```python
from build123d import *

# Parameters (mm, degrees)
EXTRUDE_1_DEPTH          = 1.6
SKETCH_2_R               = 1.1
CUT_EXTRUDE_1_DEPTH      = 40.983559121
FILLET_1_R               = 1
SKETCH_4_W               = 6.5
SKETCH_4_H               = 6.5
CUT_EXTRUDE_2_DEPTH      = 40.983559121
FILLET_2_R               = 1
SKETCH_8_W               = 28.8
SKETCH_8_H               = 14.3
CUT_EXTRUDE_3_DEPTH      = 1.6
EXTRUDE_START            = -1.75
EXTRUDE_2_DEPTH          = 26.9
CUT_EXTRUDE_4_DEPTH      = 42.601502377
CUT_EXTRUDE_4_DEPTH_BACK = 42.601502377
CUT_EXTRUDE_6_DEPTH      = 42.18403817
SHELL_START              = -28.2
SHELL_3_DEPTH            = 23.3
SHELL_START_2            = -2.83732082
SHELL_3_2_DEPTH          = 1.8
FILLET_3_R               = 3
SKETCH_15_R              = 3.1
CUT_EXTRUDE_8_DEPTH      = 1.8
FILLET_5_R               = 2
CUT_EXTRUDE_9_DEPTH      = 42.18403817
CUT_EXTRUDE_START        = -1.8
CUT_EXTRUDE_10_DEPTH     = 1.8


with BuildPart() as part:
    # 草图1 → 凸台-拉伸1 (new body)
    with BuildSketch(Plane(origin=(0, 0, 0), x_dir=(1, 0, 0), z_dir=(0, 1, 0))):
        with BuildLine():
            Line((-24.25, 8.5), (-19, 8.5))
            Line((-19, 8.5), (-19, -8.5))
            Line((-19, -8.5), (-24.25, -8.5))
            Line((-24.25, -8.5), (-24.25, -28.75))
            ThreePointArc((-24.25, -28.75), (-23.371320344, -30.871320344), (-21.25, -31.75))
            Line((-21.25, -31.75), (21.25, -31.75))
            ThreePointArc((21.25, -31.75), (23.371320344, -30.871320344), (24.25, -28.75))
            Line((24.25, -28.75), (24.25, -8.5))
            Line((24.25, -8.5), (19, -8.5))
            Line((19, -8.5), (19, 8.5))
            Line((19, 8.5), (24.25, 8.5))
            Line((24.25, 8.5), (24.25, 28.75))
            ThreePointArc((24.25, 28.75), (23.371320344, 30.871320344), (21.25, 31.75))
            Line((21.25, 31.75), (-21.25, 31.75))
            ThreePointArc((-21.25, 31.75), (-23.371320344, 30.871320344), (-24.25, 28.75))
            Line((-24.25, 28.75), (-24.25, 8.5))
        make_face()
    extrude(amount=EXTRUDE_1_DEPTH)

    # 草图2 → 切除-拉伸1 (cut, through all)
    with BuildSketch(Plane(origin=(0, 1.6, 0), x_dir=(1, 0, 0), z_dir=(0, 1, 0))):
        with Locations(Location((-19.9, 27.9, 0), (0, 0, 270))):
            Circle(SKETCH_2_R)
        with Locations(Location((19.9, 27.9, 0), (0, 0, 90))):
            Circle(SKETCH_2_R)
        with Locations(Location((19.9, -27.9, 0), (0, 0, 270))):
            Circle(SKETCH_2_R)
        with Locations(Location((-19.9, -27.9, 0), (0, 0, 90))):
            Circle(SKETCH_2_R)
    extrude(amount=-CUT_EXTRUDE_1_DEPTH, mode=Mode.SUBTRACT)

    # 圆角1
    fillet_1_edges = [part.edges().sort_by_distance(p)[0] for p in [
        (19, 0.8, -8.5),
        (19, 0.8, 8.5),
        (-19, 0.8, 8.5),
        (-19, 0.8, -8.5),
    ]]
    fillet(fillet_1_edges, radius=FILLET_1_R)

    # 草图4 → 切除-拉伸2 (cut, through all)
    with BuildSketch(Plane(origin=(0, 1.6, 0), x_dir=(1, 0, 0), z_dir=(0, 1, 0))):
        with Locations((-6, -18.75)):
            Rectangle(SKETCH_4_W, SKETCH_4_H)
        with Locations((6, -18.75)):
            Rectangle(SKETCH_4_W, SKETCH_4_H)
    extrude(amount=-CUT_EXTRUDE_2_DEPTH, mode=Mode.SUBTRACT)

    # 圆角2
    fillet_2_edges = [part.edges().sort_by_distance(p)[0] for p in [
        (-2.75, 0.8, 15.5),
        (-2.75, 0.8, 22),
        (9.25, 0.8, 15.5),
        (9.25, 0.8, 22),
        (2.75, 0.8, 22),
        (2.75, 0.8, 15.5),
        (-9.25, 0.8, 22),
        (-9.25, 0.8, 15.5),
    ]]
    fillet(fillet_2_edges, radius=FILLET_2_R)

    # 草图8 → 切除-拉伸3 (cut)
    with BuildSketch(Plane(origin=(0, 1.6, 0), x_dir=(1, 0, 0), z_dir=(0, 1, 0))):
        with Locations((0, -5.55)):
            Rectangle(SKETCH_8_W, SKETCH_8_H)
    extrude(amount=-CUT_EXTRUDE_3_DEPTH, mode=Mode.SUBTRACT)

    # 草图10 → 凸台-拉伸2 (add)
    with BuildSketch(Plane(origin=(0, 0, -31.75), x_dir=(-1, 0, 0), z_dir=(0, 0, -1)).offset(EXTRUDE_START)):
        Polygon((-9, 1.6), (9, 1.6), (7, 11.6), (-7, 11.6), align=None)
    extrude(amount=-EXTRUDE_2_DEPTH)

    # 草图11 → 切除-拉伸4 (cut, two sides: drawn at the far end of the back side and taken through both)
    with BuildSketch(Plane(origin=(0, 0, 0), x_dir=(0, 0, -1), z_dir=(1, 0, 0)).offset(-CUT_EXTRUDE_4_DEPTH_BACK)):
        Polygon((6.1, 11.6), (3.1, 4.6), (3.1, 11.6), align=None)
    extrude(amount=CUT_EXTRUDE_4_DEPTH + CUT_EXTRUDE_4_DEPTH_BACK, mode=Mode.SUBTRACT)

    # 草图14 → 切除-拉伸6 (cut, through all)
    with BuildSketch(Plane(origin=(0, 1.6, 0), x_dir=(1, 0, 0), z_dir=(0, 1, 0))):
        Polygon((-9, 30), (9, 30), (11.5, 31.75), (-11.5, 31.75), align=None)
    extrude(amount=-CUT_EXTRUDE_6_DEPTH, mode=Mode.SUBTRACT)

    # 抽壳3: read off the stored shape, not the designer's step
    # 抽壳3 outline → 抽壳3 (cut)
    with BuildSketch(Plane.XY.offset(SHELL_START)):
        Polygon((-7.484352975, 0), (7.484352975, 0), (5.524352975, 9.8), (-5.524352975, 9.8), align=None)
    extrude(amount=SHELL_3_DEPTH, mode=Mode.SUBTRACT)

    # Shell 3 2 outline → Shell 3 2 (add)
    with BuildSketch(Plane(origin=(0, 0, 0), x_dir=(1, 0, 0), z_dir=(0, 0.3939192985791679, 0.9191450300180578)).offset(SHELL_START_2)):
        Polygon((6.638245748, 5.818680827), (5.524352975, 11.878076985), (-5.524352975, 11.878076985), (-6.638245748, 5.818680827), align=None)
    extrude(amount=SHELL_3_2_DEPTH)

    # 圆角3
    fillet_3_edges = [part.edges().sort_by_distance(p)[0] for p in [
        (-11.5, 0.8, -31.75),
        (11.5, 0.8, -31.75),
        (9, 0.8, -30),
        (-9, 0.8, -30),
    ]]
    fillet(fillet_3_edges, radius=FILLET_3_R)

    # 草图15 → 切除-拉伸8 (cut)
    with BuildSketch(Plane(origin=(0, 0, -30), x_dir=(-1, 0, 0), z_dir=(0, 0, -1))):
        with Locations((0, 5.1)):
            Circle(SKETCH_15_R)
    extrude(amount=-CUT_EXTRUDE_8_DEPTH, mode=Mode.SUBTRACT)

    # 圆角5
    fillet_5_edges = [part.edges().sort_by_distance(p)[0] for p in [
        (9, 1.6, -16.626473173),
        (-9, 1.6, -16.626473173),
        (7, 11.6, -18.05),
        (-7, 11.6, -18.05),
    ]]
    fillet(fillet_5_edges, radius=FILLET_5_R)

    # 草图16 → 切除-拉伸9 (cut, through all)
    with BuildSketch(Plane(origin=(0, 1.6, 0), x_dir=(1, 0, 0), z_dir=(0, 1, 0))):
        Polygon((-11.839607805, 25.75), (-11.839607805, 28.75), (-16.839607805, 22.75), (-16.839607805, 19.75), align=None)
        Polygon((-11.839607805, 20.75), (-11.839607805, 23.75), (-16.839607805, 17.75), (-16.839607805, 14.75), align=None)
        Polygon((-11.839607805, 15.75), (-11.839607805, 18.75), (-16.839607805, 12.75), (-16.839607805, 9.75), align=None)
        Polygon((-11.839607805, 10.75), (-11.839607805, 13.75), (-16.839607805, 7.75), (-16.839607805, 4.75), align=None)
    cut_extrude_9 = extrude(amount=-CUT_EXTRUDE_9_DEPTH, mode=Mode.SUBTRACT)

    # 镜向1: 切除-拉伸9 across plane
    add(cut_extrude_9.mirror(Plane(origin=(0, 0, 0), x_dir=(0, 0, 1), z_dir=(1, 0, 0))), mode=Mode.SUBTRACT)

    # 草图18 → 切除-拉伸10 (cut)
    with BuildSketch(Plane(origin=(-8.961538462, 1.792307692, 0), x_dir=(0, 0, 1), z_dir=(-0.9805806756909202, 0.19611613513818404, 0)).offset(CUT_EXTRUDE_START)):
        Polygon((-28, 2.44349167), (-26, 2.44349167), (-24, 7.44349167), (-26, 7.44349167), align=None)
        Polygon((-23, 2.44349167), (-21, 2.44349167), (-19, 7.44349167), (-21, 7.44349167), align=None)
        Polygon((-18, 2.44349167), (-16, 2.44349167), (-14, 7.44349167), (-16, 7.44349167), align=None)
        Polygon((-13, 2.44349167), (-11, 2.44349167), (-9, 7.44349167), (-11, 7.44349167), align=None)
    cut_extrude_10 = extrude(amount=CUT_EXTRUDE_10_DEPTH, mode=Mode.SUBTRACT)

    # 镜向2: 切除-拉伸10 across plane
    add(cut_extrude_10.mirror(Plane(origin=(0, 0, 0), x_dir=(0, 0, 1), z_dir=(1, 0, 0))), mode=Mode.SUBTRACT)


solid = part.part
```
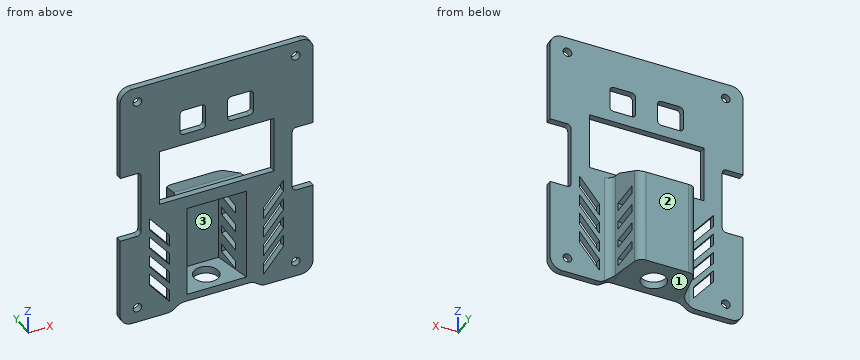
Can you work these out from the model? Positions are in its coordinate system, mm. Face numbers are marked on the shaded views. A direction names the side the tool comes from. Give positions to 0.01 mm unless a question says otherwise; leave off trailing zeros. Loops run counter-clockwise (first coordinate to the right, second up) from the corner with the lowest first, then second, coordinate; pieces in that order, holes last. Notation, with made-up numbers: M -20.5,89 L 16.5,89 A13 cw 16.5,95 Z; hole C 4.5,13.5 d1. An arc over 180 degrees is marked long. Answer in a Markdown table with one row per item.
1. Suppose I cut it at C-C on z = 11. Write out the boundary of the cut face in (x, y).
Taken from the geometry:
| item | result |
|---|---|
| outline | M -24.25,0 L -14.4,0 L -14.4,1.6 L -24.25,1.6 Z; M 14.4,0 L 24.25,0 L 24.25,1.6 L 14.4,1.6 Z |
2. For pin 1 Ø1.5 at (x, y) = (7.5, 3.5) entering from -Z; pin 2 Ø1.5 at (y, z) = (7.5, -13.5) entering from -X; pin 3 Ø1.3 at (y, z) = (0.5, -7) entering from +X; pin 4 Ø1.3 at (x, y) = (21.5, 1) entering from +Z, each with a flat end and sliding along its axis, tell me the tip position at first contact or that it passes through.
Taken from the geometry:
| item | result |
|---|---|
| pin 1 | stops at z = -30.01 |
| pin 2 | stops at x = -7.97 |
| pin 3 | stops at x = 19.01 |
| pin 4 | stops at z = 31.75 |
3. If I drill on line 1 along X through (y, z) = (1, 27.9); line 2 along Z through (x, y) = (5, 3.25); line 3 along Z through (x, y) = (6, 1.25), over which ranges is the centre line in solid material (lowest first)?
Taken from the geometry:
| item | result |
|---|---|
| line 1 | x = -24.25 to -21, -18.8 to 18.8, 21 to 24.25 |
| line 2 | z = -30 to -28.2, -4.9 to -3.1 |
| line 3 | z = -30 to -28.2, -4.9 to -1.6, 12.7 to 15.5, 22 to 31.75 |
4. Which directions (+Z, -Z, +X, -X, +Y, -Y) give clear straight access to the entire face, cutting with the end or side of a thin tool? Please do the marked faces 1, 2 and 3.
Taken from the geometry:
| item | result |
|---|---|
| face 1 | -Z, +Y, -Y |
| face 2 | +Z, -Z, +X, -X, +Y |
| face 3 | -Y |
5. Suppose I cut it at A-A on z = 18.5. Write out the boundary of the cut face in (x, y).
Taken from the geometry:
| item | result |
|---|---|
| outline | M -24.25,0 L -9.25,0 L -9.25,1.6 L -24.25,1.6 Z; M -2.75,0 L 2.75,0 L 2.75,1.6 L -2.75,1.6 Z; M 9.25,0 L 24.25,0 L 24.25,1.6 L 9.25,1.6 Z |
6. Suppose I cut it at D-D on x = 13.5. Write out the boundary of the cut face in (y, z).
Taken from the geometry:
| item | result |
|---|---|
| outline | M 0,-31.75 L 1.6,-31.75 L 1.6,-26.76 L 0,-26.76 Z; M 0,-23.76 L 1.6,-23.76 L 1.6,-21.76 L 0,-21.76 Z; M 0,-18.76 L 1.6,-18.76 L 1.6,-16.76 L 0,-16.76 Z; M 0,-13.76 L 1.6,-13.76 L 1.6,-11.76 L 0,-11.76 Z; M 0,-8.76 L 1.6,-8.76 L 1.6,-1.6 L 0,-1.6 Z; M 0,12.7 L 1.6,12.7 L 1.6,31.75 L 0,31.75 Z |
7. Suppose I cut it at B-B on x = 0. Write out the boundary of the cut face in (y, z), plus the area to 3 significant figures.
Taken from the geometry:
| item | result |
|---|---|
| outline | M 0,-30 L 2,-30 L 2,-28.2 L 0,-28.2 Z; M 0,-4.9 L 4.23,-4.9 L 9.8,-7.29 L 9.8,-28.2 L 8.2,-28.2 L 8.2,-30 L 11.6,-30 L 11.6,-6.1 L 4.6,-3.1 L 1.6,-3.1 L 1.6,-1.6 L 0,-1.6 Z; M 0,12.7 L 1.6,12.7 L 1.6,31.75 L 0,31.75 Z |
| area | 102 mm² |
